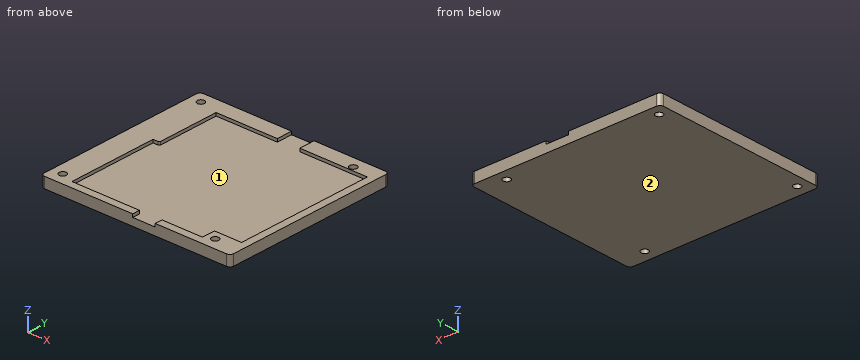
Autodesk Fusion 360 part; units mm, degrees
ref_plane "WorkPlane1" through (0, 0, 7) normal (0, 0, 1) x (1, 0, 0)
sketch "Base Plate Sketch" plane through (0, 0, 0) normal (0, 0, 1) x (1, 0, 0)
  line L0 (-58.1813, -58.7567) -> (67.977, -58.7567)
  line L1 (67.977, -58.7567) -> (67.977, 58.1813)
  line L2 (67.977, 58.1813) -> (-58.1813, 58.1813)
  line L3 (-58.1813, 58.1813) -> (-58.1813, -58.7567)
extrude "Base Plate" add sketch "Base Plate Sketch" along normal blind 7
fillet "Fillet1" radius 2.5 4 edges at (-58.1813, 58.1813, 3.5) (67.977, 58.1813, 3.5) (67.977, -58.7567, 3.5) (-58.1813, -58.7567, 3.5)
sketch "Wafer Nest Pocket Sketch" plane through (0, 0, 7) normal (0, 0, 1) x (1, 0, 0)
  line L0 (-42.023, -53.7567) -> (62.977, -53.7567)
  line L1 (62.977, -53.7567) -> (62.977, 47.704)
  line L2 (62.977, 47.704) -> (-42.023, 47.704)
  line L3 (-42.023, 47.704) -> (-42.023, -53.7567)
extrude "Wafer Nest Pocket" cut sketch "Wafer Nest Pocket Sketch" against normal blind 2
sketch "Front-Center Access Relief Sketch" plane through (0, 0, 7) normal (0, 0, 1) x (1, 0, 0)
  line L0 (2.977, -59.7567) -> (17.977, -59.7567)
  line L1 (17.977, -59.7567) -> (17.977, -50.7567)
  line L2 (17.977, -50.7567) -> (2.977, -50.7567)
  line L3 (2.977, -50.7567) -> (2.977, -59.7567)
extrude "Front-Center Access Relief" cut sketch "Front-Center Access Relief Sketch" against normal blind 2
sketch "Rear-Center Access Relief Sketch" plane through (0, 0, 7) normal (0, 0, 1) x (1, 0, 0)
  line L0 (2.977, 44.704) -> (17.977, 44.704)
  line L1 (17.977, 44.704) -> (17.977, 59.1812)
  line L2 (17.977, 59.1812) -> (2.977, 59.1812)
  line L3 (2.977, 59.1812) -> (2.977, 44.704)
extrude "Rear-Center Access Relief" cut sketch "Rear-Center Access Relief Sketch" against normal blind 2
sketch "X Datum Square Sketch (165 deg / 9:30)" plane through (0, 0, 7) normal (0, 0, 1) x (1, 0, 0)
  line L0 (-45.7852, 13.9038) -> (-37.7852, 13.9038)
  line L1 (-37.7852, 13.9038) -> (-37.7852, 6.9038)
  arc A0 (-38.7852, 5.9038) -> (-37.7852, 6.9038) centre (-38.7852, 6.9038) ccw
  line L2 (-38.7852, 5.9038) -> (-45.7852, 5.9038)
  line L3 (-45.7852, 5.9038) -> (-45.7852, 13.9038)
extrude "X Datum Square (165 deg / 9:30, rounded corner)" add sketch "X Datum Square Sketch (165 deg / 9:30)" against normal blind 2
sketch "Left Wall Flush Above X-Datum Sketch" plane through (0, 0, 7) normal (0, 0, 1) x (1, 0, 0)
  line L0 (-42.023, 13.9038) -> (-37.7852, 13.9038)
  line L1 (-37.7852, 13.9038) -> (-37.7852, 47.704)
  line L2 (-37.7852, 47.704) -> (-42.023, 47.704)
  line L3 (-42.023, 47.704) -> (-42.023, 13.9038)
extrude "Left Wall Flush Above X-Datum" add sketch "Left Wall Flush Above X-Datum Sketch" against normal blind 2
sketch "Front-Right Corner Clip (dowel) Sketch" plane through (0, 0, 7) normal (0, 0, 1) x (1, 0, 0)
  line L0 (44.9187, -53.7567) -> (62.977, -53.7567)
  line L1 (62.977, -53.7567) -> (62.977, -44.9187)
  line L2 (62.977, -44.9187) -> (44.9187, -44.9187)
  line L3 (44.9187, -44.9187) -> (44.9187, -53.7567)
extrude "Front-Right Corner Clip (dowel)" add sketch "Front-Right Corner Clip (dowel) Sketch" against normal blind 2
sketch "Outer Front Left Dowel Bore Sketch" plane through (0, 0, 7) normal (0, 0, 1) x (1, 0, 0)
  circle A0 centre (-50.8, -50.8) radius 2.3813
extrude "Outer Front Left Dowel Bore" cut sketch "Outer Front Left Dowel Bore Sketch" against normal blind 7
sketch "Outer Front Right Dowel Bore Sketch" plane through (0, 0, 7) normal (0, 0, 1) x (1, 0, 0)
  circle A0 centre (50.8, -50.8) radius 2.3813
extrude "Outer Front Right Dowel Bore" cut sketch "Outer Front Right Dowel Bore Sketch" against normal blind 7
sketch "Outer Rear Left Dowel Bore Sketch" plane through (0, 0, 7) normal (0, 0, 1) x (1, 0, 0)
  circle A0 centre (-50.8, 50.8) radius 2.3813
extrude "Outer Rear Left Dowel Bore" cut sketch "Outer Rear Left Dowel Bore Sketch" against normal blind 7
sketch "Outer Rear Right Dowel Bore Sketch" plane through (0, 0, 7) normal (0, 0, 1) x (1, 0, 0)
  circle A0 centre (50.8, 50.8) radius 2.3813
extrude "Outer Rear Right Dowel Bore" cut sketch "Outer Rear Right Dowel Bore Sketch" against normal blind 7
equation "gridPitch = 25.4 mm"
equation "indexMove = 50.8 mm"
equation "outerPinPatternSpan = 101.6 mm"
equation "dowelDiameter = 4.7625 mm"
equation "dowelHoleDiameter = 4.7625 mm"
equation "plateEdgeMargin = 5.0 mm"
equation "plateWidth = 126.15825000000001 mm"
equation "plateHeight = 116.93795079844435 mm"
equation "baseThickness = 7.0 mm"
equation "pocketDepth = 2.0 mm"
equation "nestClearanceSide = 2.5 mm"
equation "nestClearanceRear = 4.0 mm"
equation "filletRadius = 2.5 mm"
equation "primaryFlatClearance = 0.175 mm"
equation "xDatumSize = 8.0 mm"
equation "nestReliefWidth = 15.0 mm"
equation "nestOffsetX = 7.29 mm"
equation "nestOffsetY = -4.95 mm"
Read the model definition and answer for the solid it produces. Units are mm, in the model's axes. Face numbers are marked on the shaded views. Coordinates: 2 decimals unless noted, no trailing zeros. Write each loop counter-clockwise with the first axis right and the second up, starting at its lowest first coordinate (ties: lowest second). Pieces come first, ordered by that corner, then holes. Notation, with made-up numbers: (-31, 45.25) -> (9, 45.25) arc R29 ccw to (9, 69.25) -> close; hole circle Ø5 at (-16, 64). An arc over 180 degrees is marked (long way). Return JSON: item names as keys, results as strings.
(1) The part is cut by section D-D on x = -33. Give the vertices of the cut face in (y, z), then the cut area to 3 significant figures.
Answers below:
{"outline": "(-58.76, 0) -> (58.18, 0) -> (58.18, 7) -> (47.7, 7) -> (47.7, 5) -> (-53.76, 5) -> (-53.76, 7) -> (-58.76, 7) -> close", "area": "616 mm^2"}
(2) The part is cut by section C-C on y = 36. Give the vertices of the cut face in (x, z), then the cut area to 3 significant figures.
Answers below:
{"outline": "(-58.18, 0) -> (67.98, 0) -> (67.98, 7) -> (62.98, 7) -> (62.98, 5) -> (-37.79, 5) -> (-37.79, 7) -> (-58.18, 7) -> close", "area": "682 mm^2"}
(3) The part is cut by section B-B on y = -50.8. Give the vertices of the cut face in (x, z), then the cut area to 3 significant figures.
Answers below:
{"outline": "(-58.18, 0) -> (-53.18, 0) -> (-53.18, 7) -> (-58.18, 7) -> close; (-48.42, 0) -> (48.42, 0) -> (48.42, 7) -> (44.92, 7) -> (44.92, 5) -> (-42.02, 5) -> (-42.02, 7) -> (-48.42, 7) -> close; (53.18, 0) -> (67.98, 0) -> (67.98, 7) -> (53.18, 7) -> close", "area": "643 mm^2"}
(4) This flat-tipped pin is pushed along its axis until it touches: P1, Ø8, axis at x = 23, y = -12.5, coming from the +Z side. Where does it stop, or does it pass through?
Answers below:
{"P1": "z = 5"}
(5) The part is cut by section A-A on x = 50.8. Give the vertices of the cut face in (y, z).
Answers below:
{"outline": "(-58.76, 0) -> (-53.18, 0) -> (-53.18, 7) -> (-58.76, 7) -> close; (-48.42, 0) -> (48.42, 0) -> (48.42, 7) -> (47.7, 7) -> (47.7, 5) -> (-44.92, 5) -> (-44.92, 7) -> (-48.42, 7) -> close; (53.18, 0) -> (58.18, 0) -> (58.18, 7) -> (53.18, 7) -> close"}
(6) For a pull along Y with two mould halves and no side action, classify the marked faces 1 and 2 as pulls with the +Y half, pulls with the -Y half, needs draft (parallel to the pull), parting line crosses it, or undercut.
Answers below:
{"face 1": "undercut", "face 2": "needs draft"}
(7) Consider line 1 along X through (y, z) = (20, 6.5); line 2 along Z through (x, y) = (38, 27). Determine where each line is inside the solid, lowest interval first. Write a range as from..to.
Answers below:
{"line 1": "-58.18..-37.79, 62.98..67.98", "line 2": "0..5"}
